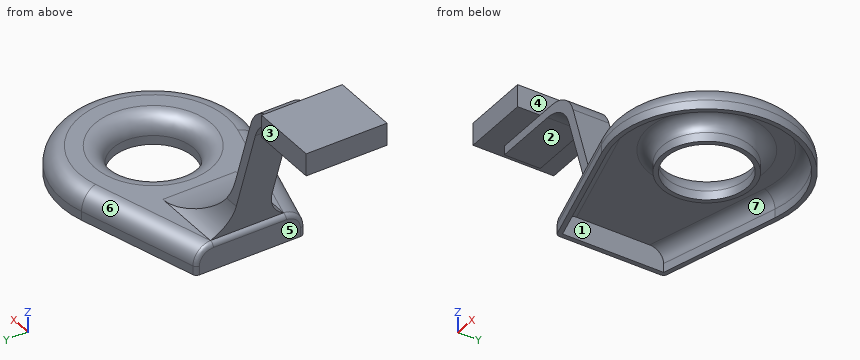
from build123d import *

# Parameters (mm, degrees)
SKETCH_R     = 20
PAD_DEPTH    = 10
FILLET_R     = 6
THICKNESS_T  = 2
PAD001_DEPTH = 20
POCKET_DEPTH = 124.001
SKETCH003_W  = 30
SKETCH003_H  = 36
PAD002_DEPTH = 10


with BuildPart() as part:
    # Sketch → Pad (new body)
    with BuildSketch(Plane.XY):
        with BuildLine():
            ThreePointArc((-10.749857, -37.489206), (39, 0), (-10.749857, 37.489206))
            Line((-10.749857, 37.489206), (-63, 22.506719))
            Line((-63, 22.506719), (-63, -22.506719))
            Line((-63, -22.506719), (-10.749857, -37.489206))
        make_face()
        Circle(SKETCH_R, mode=Mode.SUBTRACT)
    extrude(amount=PAD_DEPTH)

    # Fillet
    fillet_edges = [part.edges().sort_by_distance(p)[0] for p in [
        (-36.874928, -29.997962, 10),
        (39, 0, 10),
        (-36.874928, 29.997962, 10),
        (-20, 0, 10),
    ]]
    fillet(fillet_edges, radius=FILLET_R)

    # Thickness
    thickness_openings = [part.faces().sort_by_distance(p)[0] for p in [
        (-14.455542, 0, 0),
    ]]
    offset(amount=THICKNESS_T, openings=thickness_openings)

    # Sketch001 → Pad001 (join, symmetric)
    with BuildSketch(Plane.XZ):
        with BuildLine():
            Line((-63, 12), (-80.75207, 66.635255))
            ThreePointArc((-80.75207, 66.635255), (-86.201139, 74.135255), (-95.017918, 77))
            Line((-95.017918, 77), (-124, 77))
            Line((-124, 77), (-124, 81))
            Line((-124, 81), (-92.111748, 81))
            ThreePointArc((-77.8459, 70.635255), (-83.294969, 78.135255), (-92.111748, 81))
            Line((-77.8459, 70.635255), (-67.383016, 38.433809))
            ThreePointArc((-67.383016, 38.433809), (-53.485941, 19.306125), (-31, 12))
            Line((-63, 12), (-31, 12))
        make_face()
    extrude(amount=PAD001_DEPTH, both=True)

    # Sketch002 → Pocket (cut, through all)
    with BuildSketch(Plane.YZ):
        with BuildLine():
            Line((8, 94.265679), (8, 27.140286))
            ThreePointArc((8, 27.140286), (10.200769, 18.515653), (16.264922, 12))
            Line((16.264922, 12), (86.307831, 12))
            Line((86.307831, 124.281616), (86.307831, 12))
            Line((-95.791176, 124.281616), (86.307831, 124.281616))
            Line((-95.791176, 12), (-95.791176, 124.281616))
            Line((-16.264922, 12), (-95.791176, 12))
            ThreePointArc((-16.264922, 12), (-10.200769, 18.515653), (-8, 27.140286))
            Line((-8, 27.140286), (-8, 94.265679))
            Line((-8, 94.265679), (8, 94.265679))
        make_face()
    extrude(amount=-POCKET_DEPTH, mode=Mode.SUBTRACT)

    # Sketch003 (on Face43 of Pocket) → Pad002 (join)
    with BuildSketch(Plane.XY.offset(81)):
        with Locations((-115, 0)):
            Rectangle(SKETCH003_W, SKETCH003_H)
    extrude(amount=PAD002_DEPTH)


solid = part.part
Read the model definition and answer for the solid it produces. Units are mm, in the model's axes. Face numbers are marked on the shaded views. A direction names the side the tool comes from. Round coordinates to 2 decimals unless told otherwise and drop trailing zeros. Write each loop counter-clockwise with the first axis right and the second up, starting at its lowest first coordinate (ties: lowest second). Pieces come first, ordered by that corner, then holes. Notation, with made-up numbers: M 12.5,86.25 L 70.5,86.25 A30 cw 70.5,123.25 Z; hole C -37,-19.75 d8. An arc over 180 degrees is marked long. Use a Markdown table: item, result.
1) For a pull along Y with two mould halves and no side action, classify the marked faces 1, 2 and 3 as pulls with the +Y half, pulls with the -Y half, needs draft (parallel to the pull), parting line crosses it, or undercut.
Answers follow:
| item | result |
|---|---|
| face 1 | undercut |
| face 2 | needs draft |
| face 3 | pulls with the +Y half |
2) The part is cut by section C-C (z = 52.5). Write down the section's boundary in (x, y).
Answers follow:
| item | result |
|---|---|
| outline | M -76.16,-8 L -71.95,-8 L -71.95,8 L -76.16,8 Z |
3) The part is cut by section A-A (x = -107). Write down the section's boundary in (y, z).
Answers follow:
| item | result |
|---|---|
| outline | M -18,81 L -8,81 L -8,77 L 8,77 L 8,81 L 18,81 L 18,91 L -18,91 Z |
4) Flat-ended cylindrical pins translate along their axes: pin 1 (5 mm diameter, centred on x = -113.5, z = 88, fed in from -Y); pin 2 (5 mm diameter, centred on x = -113.5, y = -1, fed in from -Z); pin 3 (1 mm diameter, centred on x = 0.5, y = 29.5, fed in from -Z). Find the tip coordinate at first contact, or state that the pin passes through.
Answers follow:
| item | result |
|---|---|
| pin 1 | stops at y = -18 |
| pin 2 | stops at z = 77 |
| pin 3 | stops at z = 10 |
5) A tool of negligible diameter and unlimited length cuts with its end or side. For the marked faces 4, 5, 6 and 7, from which of +Z, -Z, +X, -X, +Y, -Y can it reach the whole face along a straight path? Write none if from no direction.
Answers follow:
| item | result |
|---|---|
| face 4 | +Z, +X, +Y, -Y |
| face 5 | -Z, -X, +Y, -Y |
| face 6 | +Z, -X, +Y |
| face 7 | -Z |
6) Straight lines are drawn through the part: line 1 along Y through (x, z) = (0, 1.05); line 2 along Z through (x, y) = (32, 10.5); line 3 along X through (y, z) = (-17.5, 85.5). For each, find the intervals that lie inside material, in ascending order. Write a range as [from, to].
Answers follow:
| item | result |
|---|---|
| line 1 | y = [-41, -39], [-20, -18], [18, 20], [39, 41] |
| line 2 | z = [9.96, 11.97] |
| line 3 | x = [-130, -100] |
7) The part is cut by section B-B (y = 13.5). Give the number of separate pieces and of enclosed holes in the cut face, plus the area to 3 significant figures.
Answers follow:
| item | result |
|---|---|
| separate pieces | 3 |
| enclosed holes | 0 |
| area | 585 mm2 |
